Autodesk Inventor part; units mm, degrees
ref_plane "YZ Plane" through (0, 0, 0) normal (1, 0, 0) x (0, 1, 0)
ref_plane "XZ Plane" through (0, 0, 0) normal (0, 1, 0) x (-1, 0, 0)
ref_plane "XY Plane" through (0, 0, 0) normal (0, 0, 1) x (1, 0, 0)
sketch "Sketch1" plane through (0, 0, 0) normal (0, 0, 1) x (1, 0, 0)
  point P0 (0, 0)
sketch "Sketch2" plane through (0, 0, 0) normal (0, 0, 1) x (1, 0, 0)
  circle A0 centre (0, 0) radius 20
  dimension "d0" = 40
extrude "Extrusion1" add sketch "Sketch2" along normal blind 22
sketch "Sketch3" plane through (0, 0, 22) normal (0, 0, 1) x (1, 0, 0)
  circle A0 centre (0, 0) radius 16
  dimension "d3" = 32
extrude "Extrusion2" add sketch "Sketch3" along normal blind 22.5
sketch "Sketch4" plane through (0, 0, 44.5) normal (0, 0, 1) x (1, 0, 0)
  point P0 (0, 0)
sketch "Sketch5" plane through (0, 0, 0) normal (0, 0, -1) x (-1, 0, 0)
  circle A0 centre (0, 0) radius 11.25
  dimension "d8" = 22.5
extrude "Extrusion3" add sketch "Sketch5" along normal blind 9
sketch "Sketch6" plane through (0, 0, -9) normal (0, 0, -1) x (-1, 0, 0)
  circle A0 centre (0, 0) radius 2.75
  dimension "d11" = 5.5
extrude "Extrusion4" add sketch "Sketch6" along normal blind 24
properties part number "DC MOTOR 1"
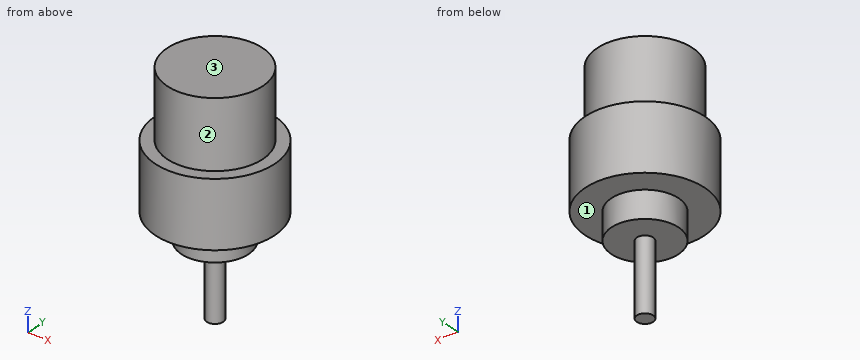
Design review of the part built by this model. Coordinates are the model's own, in mm. Face numbers are marked on the shaded views. A direction names the side the tool comes from. Round coordinates to 2 decimals unless told otherwise and drop trailing zeros. Loops run counter-clockwise (first coordinate to the right, second up) from the corner with the lowest first, then second, coordinate; pieces in that order, holes last. Notation, with made-up numbers: (78, 31.25) - (130, 31.25) arc R28 ccw to (130, 51.25) - close; hole circle Ø4 at (53.5, 24.5). An arc over 180 degrees is marked (long way). One line per question, with ' | ' between items.
1. We need section A-A, the plane y = 0. State the section outline as (x, z) points.
Results are:
outline: (-20, 0) - (-11.25, 0) - (-11.25, -9) - (-2.75, -9) - (-2.75, -33) - (2.75, -33) - (2.75, -9) - (11.25, -9) - (11.25, 0) - (20, 0) - (20, 22) - (16, 22) - (16, 44.5) - (-16, 44.5) - (-16, 22) - (-20, 22) - close
2. Clearance check with flat-ended pins moving along their axes: P1, Ø10, axis at x = -13, y = -14.5, coming from the -Z side; P2, Ø1.5, axis at y = -0.5, z = -21, coming from the +X side; P3, Ø4, axis at y = -5, z = 25, coming from the -X side. State where each tip first meets the part, or that it passes through.
Results are:
P1: stops at z = 0 | P2: stops at x = 2.75 | P3: stops at x = -15.72
3. For L1, parallel to Z at x = -12, y = 5; L2, parallel to Z at x = 13.5, y = 14; L3, parallel to Y at x = 0, z = 3, list the stretches that pass through material, from the lowest coordinate up. Write a range as [from, to].
Results are:
L1: z = [0, 44.5] | L2: z = [0, 22] | L3: y = [-20, 20]
4. We need section C-C, the plane z = 1.5. State the section outline as (x, y) points.
Results are:
outline: circle Ø40 at (0, 0)
5. We need section B-B, the plane x = -13.5. State the section outline as (y, z) points, and give its area (3 significant figures).
Results are:
outline: (-14.76, 0) - (14.76, 0) - (14.76, 22) - (8.59, 22) - (8.59, 44.5) - (-8.59, 44.5) - (-8.59, 22) - (-14.76, 22) - close | area: 1,040 mm²
6. For the marked faces 1, 2 and 3, list the 3-axis set-ups (+Z, -Z, +X, -X, +Y, -Y) from which the entire face can be reached by the end or side of a thin tool; tool diameter is ignored.
Results are:
face 1: -Z | face 2: +Z | face 3: +Z, +X, -X, +Y, -Y
